Check sheet for the modelled part. Datum: model origin and axes. Units: mm. Round coordinates to 2 decimals unless told otherwise and drop trailing zeros. Order: outer loops, then holes, each group sorted by start corner. A loop starts at its lowest first (then second) coordinate and runs counter-clockwise, first axis right, second up. Notation, with made-up numbers: (42.5, 86.25) -> (79.5, 86.25) arc R15 cw to (79.5, 103.25) -> close; hole circle Ø1 at (-33.5, -31). An arc over 180 degrees is marked (long way). Answer as CSV lines item,"result". Start each with the question number.
from build123d import *

# Parameters (mm, degrees)
SKETCH_1_R      = 30
SKETCH_1_R_2    = 22.5
SKETCH_1_R_3    = 1.6
EXTRUDE_1_DEPTH = 3
SKETCH_4_R      = 1.5
EXTRUDE_3_DEPTH = 3
FILLET_1_R      = 5
FILLET_2_R      = 5


with BuildPart() as part:
    # 草图1 → 凸台-拉伸1 (new body)
    with BuildSketch(Plane.XY):
        Circle(SKETCH_1_R)
        Circle(SKETCH_1_R_2, mode=Mode.SUBTRACT)
        with Locations((23.815698604, 13.75)):
            Circle(SKETCH_1_R_3, mode=Mode.SUBTRACT)
        with Locations((0, -27.5)):
            Circle(SKETCH_1_R_3, mode=Mode.SUBTRACT)
        with Locations((-23.815698604, 13.75)):
            Circle(SKETCH_1_R_3, mode=Mode.SUBTRACT)
    extrude(amount=EXTRUDE_1_DEPTH)

    # 草图4 → 凸台-拉伸3 (add)
    with BuildSketch(Plane.XY.offset(3)):
        with BuildLine():
            Line((-18.354989219, 23.729609579), (35, 65))
            Line((35, 65), (35, 77))
            Line((35, 77), (53, 77))
            Line((53, 77), (53, 59.959453772))
            Line((53, 59.959453772), (11.372950108, 27.760691739))
            Line((11.372950108, 27.760691739), (1.135189229, 26.37246046))
            ThreePointArc((1.135189229, 26.37246046), (-0.214991049, 29.085490097), (-0.793931536, 26.110873398))
            Line((-0.793931536, 26.110873398), (-18.354989219, 23.729609579))
        make_face()
        with Locations((40, 70.2)):
            Circle(SKETCH_4_R, mode=Mode.SUBTRACT)
        with Locations((48, 70.2)):
            Circle(SKETCH_4_R, mode=Mode.SUBTRACT)
    extrude(amount=-EXTRUDE_3_DEPTH)

    # 圆角1
    fillet_1_edges = [part.edges().sort_by_distance(p)[0] for p in [
        (11.372950108, 27.760691739, 1.5),
    ]]
    fillet(fillet_1_edges, radius=FILLET_1_R)

    # 圆角2
    fillet_2_edges = [part.edges().sort_by_distance(p)[0] for p in [
        (35, 65, 1.5),
        (53, 59.959453772, 1.5),
    ]]
    fillet(fillet_2_edges, radius=FILLET_2_R)


solid = part.part
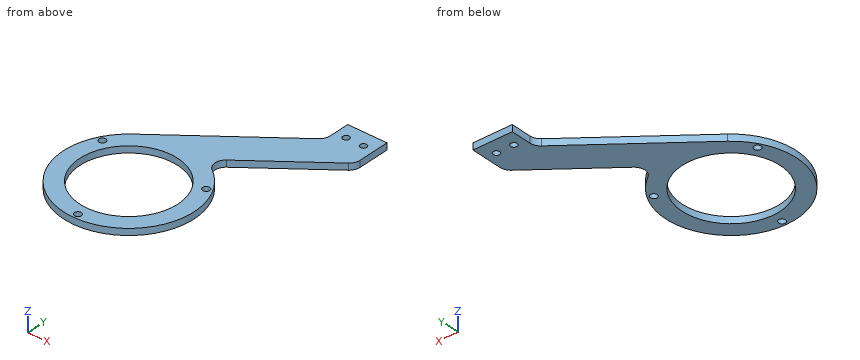
1) Material ranges on line 1 along X through (y, z) = (70.2, 0.65); line 2 along Y through (x, z) = (-13, 0.85); line 3 along X through (y, z) = (-6, 2.7), recorded low to high.
2) Section check D-D on y = 70.2. Record the cut outline in (x, z), then the cut area to 3 significant figures.
3) Section check B-B on z = 0.7. Record the cut outline in (x, y).
4) Section check A-A on y = 0. Record the cut outline in (x, z), then the cut area to 3 significant figures.
5) Section check C-C on x = 40. Record the cut outline in (y, z).
Solutions:
1,line 1,"x = 35 to 38.5, 41.5 to 46.5, 49.5 to 53"
1,line 2,"y = -27.04 to -18.36, 18.36 to 27.87"
1,line 3,"x = -29.39 to -21.69, 21.69 to 29.39"
2,outline,"(35, 0) -> (38.5, 0) -> (38.5, 3) -> (35, 3) -> close; (41.5, 0) -> (46.5, 0) -> (46.5, 3) -> (41.5, 3) -> close; (49.5, 0) -> (53, 0) -> (53, 3) -> (49.5, 3) -> close"
2,area,"36.0 mm^2"
3,outline,"(-18.35, 23.73) arc R30 ccw (long way) to (17.5, 24.37) arc R5 cw to (17.35, 32.39) -> (51.06, 58.46) arc R5 ccw to (53, 62.41) -> (53, 77) -> (35, 77) -> (35, 67.45) arc R5 cw to (33.06, 63.5) -> close; hole circle Ø3.2 at (-23.82, 13.75); hole circle Ø45 at (0, 0); hole circle Ø3.2 at (0, -27.5); hole circle Ø3.2 at (23.82, 13.75); hole circle Ø3 at (40, 70.2); hole circle Ø3 at (48, 70.2)"
4,outline,"(-30, 0) -> (-22.5, 0) -> (-22.5, 3) -> (-30, 3) -> close; (22.5, 0) -> (30, 0) -> (30, 3) -> (22.5, 3) -> close"
4,area,"45.0 mm^2"
5,outline,"(49.9, 0) -> (68.7, 0) -> (68.7, 3) -> (49.9, 3) -> close; (71.7, 0) -> (77, 0) -> (77, 3) -> (71.7, 3) -> close"
